from build123d import *

# Parameters (mm, degrees)
ESBO_O1_W                = 120
ESBO_O1_H                = 80
ESBO_O1_R                = 1.501648648
ESBO_O1_W_2              = 40.2
ESBO_O1_H_2              = 20.2
ESBO_O1_W_3              = 5.5
ESBO_O1_H_3              = 4
RESSALTO_EXTRUS_O4_DEPTH = 7
RESSALTO_EXTRUS_O5_START = 7
ESBO_O1_12_W             = 57.88
ESBO_O1_12_H             = 26.2
ESBO_O1_12_R             = 1.501648648
ESBO_O1_12_W_2           = 40.2
ESBO_O1_12_H_2           = 20.2
RESSALTO_EXTRUS_O5_DEPTH = 5.58
ESBO_O9_R                = 1.6
CORTE_EXTRUS_O7_DEPTH    = 10
CORTE_EXTRUS_O8_START    = -10
ESBO_O10_R               = 1.6
CORTE_EXTRUS_O8_DEPTH    = 10


with BuildPart() as part:
    # Esboço1 → Ressalto-extrusão4 (new body)
    with BuildSketch(Plane.XY):
        Rectangle(ESBO_O1_W, ESBO_O1_H)
        with Locations((34.63, -4.9)):
            Circle(ESBO_O1_R, mode=Mode.SUBTRACT)
        with Locations((34.63, 4.9)):
            Circle(ESBO_O1_R, mode=Mode.SUBTRACT)
        with Locations((-14.17, -4.9)):
            Circle(ESBO_O1_R, mode=Mode.SUBTRACT)
        with Locations((-14.17, 4.9)):
            Circle(ESBO_O1_R, mode=Mode.SUBTRACT)
        with Locations((10.23, 0)):
            Rectangle(ESBO_O1_W_2, ESBO_O1_H_2, mode=Mode.SUBTRACT)
        with Locations((-47.46, -35)):
            Rectangle(ESBO_O1_W_3, ESBO_O1_H_3, mode=Mode.SUBTRACT)
        with Locations((47.46, -35)):
            Rectangle(ESBO_O1_W_3, ESBO_O1_H_3, mode=Mode.SUBTRACT)
        with Locations((0, -35)):
            Rectangle(ESBO_O1_W_3, ESBO_O1_H_3, mode=Mode.SUBTRACT)
        with Locations((47.46, 35)):
            Rectangle(ESBO_O1_W_3, ESBO_O1_H_3, mode=Mode.SUBTRACT)
        with Locations((0, 35)):
            Rectangle(ESBO_O1_W_3, ESBO_O1_H_3, mode=Mode.SUBTRACT)
        with Locations((-47.46, 35)):
            Rectangle(ESBO_O1_W_3, ESBO_O1_H_3, mode=Mode.SUBTRACT)
    extrude(amount=RESSALTO_EXTRUS_O4_DEPTH)

    # Esboço1<12> → Ressalto-extrusão5 (add)
    with BuildSketch(Plane.XY.offset(RESSALTO_EXTRUS_O5_START)):
        with Locations((10.09, 0)):
            Rectangle(ESBO_O1_12_W, ESBO_O1_12_H)
        with Locations(Location((-14.17, 4.9, 0), (0, 0, 180))):
            Circle(ESBO_O1_12_R, mode=Mode.SUBTRACT)
        with Locations(Location((34.63, 4.9, 0), (0, 0, 180))):
            Circle(ESBO_O1_12_R, mode=Mode.SUBTRACT)
        with Locations(Location((34.63, -4.9, 0), (0, 0, 180))):
            Circle(ESBO_O1_12_R, mode=Mode.SUBTRACT)
        with Locations(Location((-14.17, -4.9, 0), (0, 0, 180))):
            Circle(ESBO_O1_12_R, mode=Mode.SUBTRACT)
        with Locations((10.23, 0)):
            Rectangle(ESBO_O1_12_W_2, ESBO_O1_12_H_2, mode=Mode.SUBTRACT)
    extrude(amount=RESSALTO_EXTRUS_O5_DEPTH)

    # Esboço9 → Corte-extrusão7 (cut)
    with BuildSketch(Plane.XZ.offset(40)):
        with Locations(Location((-47.46, 3.5, 0), (0, 0, 270))):
            Circle(ESBO_O9_R)
        with Locations(Location((0, 3.5, 0), (0, 0, 270))):
            Circle(ESBO_O9_R)
        with Locations((47.46, 3.5)):
            Circle(ESBO_O9_R)
    extrude(amount=-CORTE_EXTRUS_O7_DEPTH, mode=Mode.SUBTRACT)

    # Esboço10 → Corte-extrusão8 (cut)
    with BuildSketch(Plane(origin=(0, 40, 0), x_dir=(1, 0, 0), z_dir=(0, 1, 0)).offset(CORTE_EXTRUS_O8_START)):
        with Locations(Location((-47.46, -3.5, 0), (0, 0, 90))):
            Circle(ESBO_O10_R)
        with Locations(Location((0, -3.5, 0), (0, 0, 90))):
            Circle(ESBO_O10_R)
        with Locations((47.46, -3.5)):
            Circle(ESBO_O10_R)
    extrude(amount=CORTE_EXTRUS_O8_DEPTH, mode=Mode.SUBTRACT)


solid = part.part
Model file for the job. Use its own axes, mm. A direction names the side the tool comes from. Coordinates: 2 decimals unless noted, no trailing zeros. Write each loop counter-clockwise with the first axis right and the second up, starting at its lowest first coordinate (ties: lowest second). Pieces come first, ordered by that corner, then holes. Notation, with made-up numbers: (21.5, 49) - (46.5, 49) arc R29 ccw to (46.5, 85) - close; hole circle Ø1 at (51, -26). An arc over 180 degrees is marked (long way). Write each question's results on one line, items separated by ' | '. Start each with the question number.
1) Probe line 1 along X through (y, z) = (32.25, 3.5); line 2 along X through (y, z) = (4.9, 6.5); line 3 along Y through (x, z) = (-7, 8.5). List the from-to ranges inside material, lowest first. Write a range as from..to.
2) Cut at C-C (x = -47.46). Write the cut outline in (y, z).
3) Cut at B-B (z = 9). Write the cut outline in (x, y), then the cut area to 3 significant figures.
4) Cut at A-A (x = 6.5). Write the cut outline in (y, z).
5) Flat gauge pins, fed straight in: P1, Ø2, axis at x = 3, z = 10.5, coming from the -Y side; P2, Ø1.5, axis at x = 47, y = -2.5, coming from the +Z side; P3, Ø1.9, axis at x = 47.46, z = 3.5, coming from the +Y side; P4, Ø2.5, axis at x = -14.17, y = -4.9, coming from the -Z side. Where does each tip first touch, or does it go through?
6) 3-axis set-ups, long thin cutter, end or side, ignore diameter. For faces 1 (the face through (-0.61, -38.52, 2.02)), 2 (the face through (45.6, -37, 3.5)), 3 (the face through (-18.85, 0, 10)), 4 (the face through (-47, 30, 4)): which of +Z, -Z, +X, -X, +Y, -Y reach the whole face in a straight line?
7) Mould opens along Z. For faces 5 (the face through (-45.7, 37, 3.5)), 6 (the face through (-46.11, -38.52, 2.64)) say: pulls with the +Z half, pulls with the -Z half, needs draft (parallel to the pull), parting line crosses it, or undercut.
Returned:
1) line 1: -60..-49.06, -45.86..-1.6, 1.6..45.86, 49.06..60 | line 2: -60..-15.67, -12.67..-9.87, 30.33..33.13, 36.13..60 | line 3: -13.1..-10.1, 10.1..13.1
2) outline: (-40, 0) - (-37, 0) - (-37, 1.9) - (-40, 1.9) - close; (-40, 5.1) - (-37, 5.1) - (-37, 7) - (-40, 7) - close; (-33, 0) - (33, 0) - (33, 1.9) - (30, 1.9) - (30, 5.1) - (33, 5.1) - (33, 7) - (-33, 7) - (-33, 5.1) - (-30, 5.1) - (-30, 1.9) - (-33, 1.9) - close; (37, 0) - (40, 0) - (40, 1.9) - (37, 1.9) - close; (37, 5.1) - (40, 5.1) - (40, 7) - (37, 7) - close
3) outline: (-18.85, -13.1) - (39.03, -13.1) - (39.03, 13.1) - (-18.85, 13.1) - close; hole circle Ø3 at (-14.17, -4.9); hole circle Ø3 at (-14.17, 4.9); hole (-9.87, -10.1) - (30.33, -10.1) - (30.33, 10.1) - (-9.87, 10.1) - close; hole circle Ø3 at (34.63, -4.9); hole circle Ø3 at (34.63, 4.9) | area: 676 mm^2
4) outline: (-40, 0) - (-10.1, 0) - (-10.1, 12.58) - (-13.1, 12.58) - (-13.1, 7) - (-40, 7) - close; (10.1, 0) - (40, 0) - (40, 7) - (13.1, 7) - (13.1, 12.58) - (10.1, 12.58) - close
5) P1: y = -13.1 | P2: z = 7 | P3: y = 30 | P4: through
6) face 1: -Y | face 2: +Z, -Z | face 3: +Z, -X, +Y, -Y | face 4: +Y
7) face 5: needs draft | face 6: undercut
